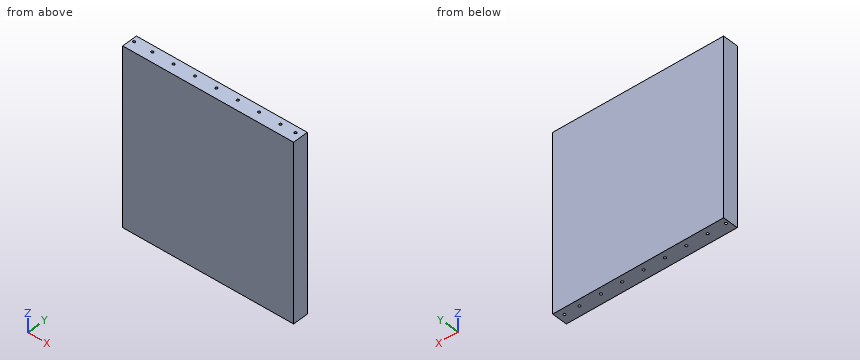
```python
from build123d import *

# Parameters (mm, degrees)
SKETCH1_W           = 2032
SKETCH1_H           = 184.15
BOSS_EXTRUDE1_DEPTH = 2108.2
SKETCH2_R           = 14.2875
CUT_EXTRUDE1_DEPTH  = 2934.844314632


with BuildPart() as part:
    # Sketch1 → Boss-Extrude1 (new body)
    with BuildSketch(Plane.XY):
        with Locations((1016, 92.075)):
            Rectangle(SKETCH1_W, SKETCH1_H)
    extrude(amount=BOSS_EXTRUDE1_DEPTH)

    # Sketch2 → Cut-Extrude1 (cut, through all)
    with BuildSketch(Plane.XY):
        with Locations((38.1, 111.125)):
            Circle(SKETCH2_R)
        with Locations((254, 111.125)):
            Circle(SKETCH2_R)
        with Locations((508, 111.125)):
            Circle(SKETCH2_R)
        with Locations((762, 111.125)):
            Circle(SKETCH2_R)
        with Locations((1016, 111.125)):
            Circle(SKETCH2_R)
        with Locations((1270, 111.125)):
            Circle(SKETCH2_R)
        with Locations((1524, 111.125)):
            Circle(SKETCH2_R)
        with Locations((1778, 111.125)):
            Circle(SKETCH2_R)
        with Locations((1955.8, 111.125)):
            Circle(SKETCH2_R)
    extrude(amount=CUT_EXTRUDE1_DEPTH, mode=Mode.SUBTRACT)


solid = part.part
```
Read the model definition and answer for the solid it produces. Units are mm, in the model's axes. Round coordinates to 2 decimals unless told otherwise and drop trailing zeros. One line per item, written item: value.
Q1. Straight lines are drawn through the part: line 1 (Y direction, x = 1016, z = 625); line 2 (Y direction, x = 763.5, z = 1126.5). For each, find the intervals that lie inside material, in ascending order. Write a range as [from, to].
Data:
line 1: [0, 96.84], [125.41, 184.15]
line 2: [0, 96.92], [125.33, 184.15]
Q2. A flat-ended cylindrical pin translates along its axis: pin 1 Ø23 at (x, y) = (38.1, 111.125) entering from -Z. Find the tip coordinate at first contact, or state that the pin passes through.
Data:
pin 1: through
Q3. Find section A-A on z = 548. Count the separate pieces of the cut face and the enclosed holes in it, plus the area to 3 significant figures.
Data:
separate pieces: 1
enclosed holes: 9
area: 368,000 mm2
